Verification items for the finished model (mm, model axes). A direction names the side the tool comes from. Round coordinates to 2 decimals unless told otherwise and drop trailing zeros. Order: outer loops, then holes, each group sorted by start corner. A loop starts at its lowest first (then second) coordinate and runs counter-clockwise, first axis right, second up. Notation, with made-up numbers: M 45,10 L 61,10 A11 cw 61,26 Z; hole C -19,78 d11. An arc over 180 degrees is marked long. Use CSV: the item, a comma, the result in double quotes. Start each with the question number.
Q1. Scan lines: line 1 (X direction, y = 0, z = -23.9) (3 decimals); line 2 (Z direction, x = 0, y = -14); line 3 (Y direction, x = -60, z = 20.5). Record each from-to range of solid material in increasing order.
Q2. Gauge pin test, flat ends, axial feed: pin 1 Ø7 at (y, z) = (-3, -16) entering from +X; pin 2 Ø3.5 at (x, z) = (-94, -24.5) entering from +Y; pin 3 Ø18.5 at (y, z) = (-2.5, -10.5) entering from -X. Record the tip position at first contact, or that the pin passes through.
Q3. Sectioned sample at A-A (z = -3.5). Enter the section's corners in (x, y).
Q4. Mould release check, pull along Z, two halves, no side actions. Record for faces 1 (the face through (103.25, -17.6, -24.56)), 2 (the face through (-89, 0, -26.167)), 3 (the face through (76.2, 0, -11)): +Z half, -Z half, draft (parallel to the pull), parting line (faces both ways), or undercut.
Q5. Set-up check for faces 4 (the face through (-55, -12.7, 11)), 5 (the face through (55, 12.7, 14)), 6 (the face through (88.9, 0, -12)), 7 (the face through (-55, 12.7, 11)): record each of +Z, -Z, +X, -X, +Y, -Y from which the full face is reachable in a straight line by a thin tool's end or side.
```python
from build123d import *

# Parameters (mm, degrees)
F0_R     = 26
F1_DEPTH = 25.4
F2_DEPTH = 12.7
F3_W     = 31.75
F3_H     = 38.1
F4_DEPTH = 3.175
F5_R     = 5.08
F6_R     = 5.08
F7_R     = 2.5
F8_DEPTH = 25.4


with BuildPart() as f1:
    # F0 (on Front) → F1 (new body, symmetric)
    with BuildSketch(Plane.XZ):
        with BuildLine():
            ThreePointArc((1.10512, 21.131636), (21.600389, 30.292455), (30, 51.111274))
            ThreePointArc((30, 51.111274), (0, 81.111274), (-30, 51.111274))
            ThreePointArc((-30, 51.111274), (-21.605128, 30.297373), (-1.11877, 21.132142))
            add(Edge.make_bspline(
                [(-1.11877, 21.132142), (-0.729546, 21.131124), (-0.356346, 21.124225), (0, 21.111274)],
                knots=[77.429523, 77.429523, 77.429523, 77.429523, 79.070386, 79.070386, 79.070386, 79.070386], degree=3))
            add(Edge.make_bspline(
                [(1.10512, 21.131636), (0.702299, 21.134485), (0.333214, 21.127816), (0, 21.111274)],
                knots=[76.974546, 76.974546, 76.974546, 76.974546, 79.070386, 79.070386, 79.070386, 79.070386], degree=3))
        make_face()
        with Locations((0, 51.111274)):
            Circle(F0_R, mode=Mode.SUBTRACT)
    extrude(amount=F1_DEPTH, both=True)

    # F0 (on Front) → F2 (join, symmetric)
    with BuildSketch(Plane.XZ):
        with BuildLine():
            ThreePointArc((-1.11877, 21.132142), (-21.605128, 30.297373), (-30, 51.111274))
            add(Edge.make_bspline(
                [(-30, 51.111274), (-30, 18.52078), (-88.9, 22.936654), (-88.9, 0)],
                knots=[0, 0, 0, 0, 77.984436, 77.984436, 77.984436, 77.984436], degree=3))
            Line((-88.9, 0), (-88.9, -26.166598))
            Line((-88.9, -26.166598), (-76.2, -26.166598))
            Line((-76.2, -26.166598), (-76.2, 0))
            add(Edge.make_bspline(
                [(-76.2, 0), (-73.534535, 8.132415), (-19.485583, 21.180166), (-1.11877, 21.132142)],
                knots=[0, 0, 0, 0, 77.429523, 77.429523, 77.429523, 77.429523], degree=3))
        make_face()
        with BuildLine():
            add(Edge.make_bspline(
                [(30, 51.111274), (30, 18.52078), (88.9, 22.936654), (88.9, 0)],
                knots=[0, 0, 0, 0, 77.984436, 77.984436, 77.984436, 77.984436], degree=3))
            ThreePointArc((30, 51.111274), (21.600389, 30.292455), (1.10512, 21.131636))
            add(Edge.make_bspline(
                [(76.2, 0), (76.2, 8.084629), (15.899645, 21.026998), (1.10512, 21.131636)],
                knots=[0, 0, 0, 0, 76.974546, 76.974546, 76.974546, 76.974546], degree=3))
            Line((76.2, 0), (76.2, -26.166598))
            Line((76.2, -26.166598), (88.9, -26.166598))
            Line((88.9, -26.166598), (88.9, 0))
        make_face()
    extrude(amount=F2_DEPTH, both=True)

    # F3 (on face) → F4 (join)
    with BuildSketch(Plane(origin=(0, 0, -26.166598), x_dir=(1, 0, 0), z_dir=(0, 0, -1))):
        with Locations((-88.9, 0)):
            Rectangle(F3_W, F3_H)
        with Locations((88.9, 0)):
            Rectangle(F3_W, F3_H)
    extrude(amount=-F4_DEPTH)

    # F5
    f5_edges = [f1.edges().sort_by_distance(p)[0] for p in [
        (-104.775, -19.05, -24.579098),
        (-73.025, -19.05, -24.579098),
        (-104.775, 19.05, -24.579098),
        (-73.025, 19.05, -24.579098),
    ]]
    fillet(f5_edges, radius=F5_R)

    # F6
    f6_edges = [f1.edges().sort_by_distance(p)[0] for p in [
        (104.775, -19.05, -24.579098),
        (73.025, -19.05, -24.579098),
        (104.775, 19.05, -24.579098),
        (73.025, 19.05, -24.579098),
    ]]
    fillet(f6_edges, radius=F6_R)

    # F7 (on face) → F8 (cut)
    with BuildSketch(Plane(origin=(0, 0, -26.166598), x_dir=(1, 0, 0), z_dir=(0, 0, -1))):
        with Locations((-94.0308, 0)):
            Circle(F7_R)
        with Locations((94.017617, 0)):
            Circle(F7_R)
    extrude(amount=-F8_DEPTH, mode=Mode.SUBTRACT)


solid = f1.part
```
Verdict:
1,line 1,"x = -104.775 to -96.531, -91.531 to -73.025, 73.025 to 91.518, 96.518 to 104.775"
1,line 2,"z = 21.11 to 25.11, 77.11 to 81.11"
1,line 3,"y = -12.7 to 12.7"
2,pin 1,"stops at x = 88.9"
2,pin 2,"stops at y = 19.05"
2,pin 3,"stops at x = -88.9"
3,outline,"M -88.9,-12.7 L -76.2,-12.7 L -76.2,12.7 L -88.9,12.7 Z; M 76.2,-12.7 L 88.9,-12.7 L 88.9,12.7 L 76.2,12.7 Z"
4,face 1,"draft"
4,face 2,"-Z half"
4,face 3,"undercut"
5,face 4,"-X, -Y"
5,face 5,"+X, +Y"
5,face 6,"+Z, +X, +Y, -Y"
5,face 7,"-X, +Y"
